Could you check a few things on this model? Use its own coordinates, in mm. Face numbers are marked on the shaded views. Give positions to 0.01 mm unless a question says otherwise; leave off trailing zeros. Order: outer loops, then holes, each group sorted by start corner. A loop starts at its lowest first (then second) coordinate and runs counter-clockwise, first axis right, second up. Notation, with made-up numbers: (3.25, 12) -> (58.25, 12) arc R23 cw to (58.25, 31) -> close; hole circle Ø8 at (-19.75, -25). An arc over 180 degrees is marked (long way). One line per item, written item: value.
Autodesk Inventor part; units mm, degrees
ref_plane "YZ Plane" through (0, 0, 0) normal (1, 0, 0) x (0, 1, 0)
ref_plane "XY Plane" through (0, 0, 0) normal (0, 0, 1) x (1, 0, 0)
sketch "Sketch1" plane through (0, 0, 0) normal (0, 0, 1) x (1, 0, 0)
  line L0 (0, 0) -> (0, 13.5)
  line L1 (0, 13.5) -> (60, 13.5)
  line L2 (60, 13.5) -> (60, 0)
  line L3 (60, 0) -> (0, 0)
  line L4 (0, 0) -> (64.8862, 0) construction
  dimension "d0" = 13.5
  dimension "d1" = 60
revolve "Revolution3" add sketch "Sketch1" angle 360 about axis through (0, 0, 0) along (1, 0, 0)
ref_plane "Work Plane3" through (0, -9.5, 0) normal (0, 1, 0) x (-1, 0, 0)
sketch "Sketch5" plane through (0, -9.5, 0) normal (0, 1, 0) x (-1, 0, 0)
  line L0 (0, 0) -> (-33, 0) construction
  line L1 (-33, 0) -> (-36.5, 0) construction
  line L2 (-36.5, 0) -> (-56.5, 0) construction
  line L3 (-46.5, 0) -> (-40.5, 0)
  line L4 (-40.5, 0) -> (-52.5, 0)
  arc A0 (-40.5, -4) -> (-40.5, 4) centre (-40.5, 0) ccw
  arc A1 (-52.5, 4) -> (-52.5, -4) centre (-52.5, 0) ccw
  line L5 (-40.5, -4) -> (-52.5, -4)
  line L6 (-40.5, 4) -> (-52.5, 4)
  dimension "d39" = 33
  dimension "d40" = 3.5
  dimension "d41" = 20
  dimension "d42" = 6
  dimension "d43" = 12
  dimension "d44" = 8
  dimension "d45" = 8
sketch "Sketch6" plane through (0, 0, 0) normal (-1, 0, 0) x (0, 0, 1)
  circle A0 centre (0, 0) radius 13.5
  line L0 (0, 13.5) -> (0, -9.5)
  line L1 (0, -9.5) -> (9.5917, -9.5)
  line L2 (0, -9.5) -> (-9.5917, -9.5)
  dimension "d46" = 23
extrude "Extrusion1" cut sketch "Sketch5" against normal blind 4
thread "Thread1"
sketch "Sketch7" plane through (52.5, -9.5, 4) normal (0, 0, -1) x (-1, 0, 0)
  point P0 (52.5, 9.5)
properties part number "Cilindro Inicial con Corte" material "Aluminum 6061"
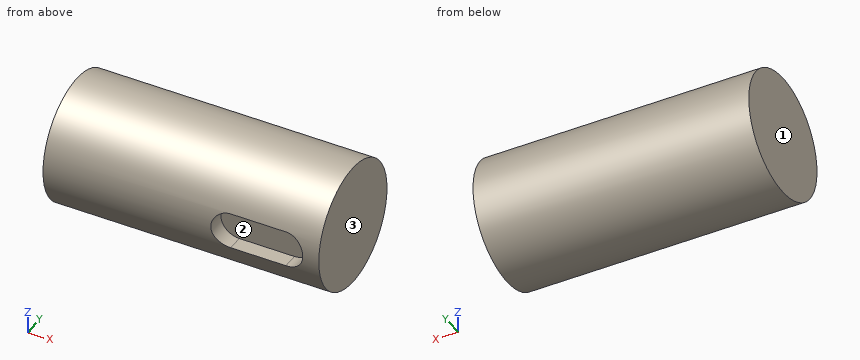
1) Suppose I cut it at B-B, the plane x = 51. Write out the boundary of the cut face in (y, z), then the cut area to 3 significant figures.
Answer below:
outline: (-12.89, -4) arc R13.5 ccw (long way) to (-12.89, 4) -> (-9.5, 4) -> (-9.5, -4) -> close
area: 542 mm2
2) Suppose I cut it at A-A, the plane z = 0. Write out the boundary of the cut face in (x, y).
Answer below:
outline: (0, -13.5) -> (36.5, -13.5) -> (36.5, -9.5) -> (56.5, -9.5) -> (56.5, -13.5) -> (60, -13.5) -> (60, 13.5) -> (0, 13.5) -> close
3) We'd pull the mould along X, two halves only. Please class the marked faces 1, 2 and 3: +X half, -X half, draft (parallel to the pull), parting line (faces both ways), or undercut.
Answer below:
face 1: -X half
face 2: undercut
face 3: +X half
4) Suppose I cut it at C-C, the plane y = -4. Write out the boundary of the cut face in (x, z), then the cut area to 3 significant figures.
Answer below:
outline: (0, -12.89) -> (60, -12.89) -> (60, 12.89) -> (0, 12.89) -> close
area: 1,550 mm2
5) For P1, Ø1, axis at x = 46.5, y = -10.5, coming from the +Z side; P2, Ø3.5, axis at x = 43.5, y = -10.5, coming from the -Z side; P3, Ø4, axis at x = 36.5, y = 3.5, coming from the -Z side, each with a flat end and sliding along its axis, tell me the tip position at first contact or that it passes through.
Answer below:
P1: stops at z = 9.07
P2: stops at z = -10.28
P3: stops at z = -13.42
6) If I drill on line 1 along Z through (x, y) = (56, -10.5); line 2 along Z through (x, y) = (39, -10.75); line 3 along Y through (x, z) = (42, -5), over which ranges is the centre line in solid material (lowest first)?
Answer below:
line 1: z = -8.49 to -1.94, 1.94 to 8.49
line 2: z = -8.17 to -3.71, 3.71 to 8.17
line 3: y = -12.54 to 12.54
7) Suppose I cut it at D-D, the plane x = 12.5. Write out the boundary of the cut face in (y, z), then the cut area to 3 significant figures.
Answer below:
outline: circle Ø27 at (0, 0)
area: 573 mm2
